Part model, mm, in its own coordinate system. Coordinates: 2 decimals unless noted, no trailing zeros. Loops run counter-clockwise (first coordinate to the right, second up) from the corner with the lowest first, then second, coordinate; pieces in that order, holes last. Notation, with made-up numbers: (60, -15.75) -> (76, -15.75) arc R20 cw to (76, -5.75) -> close; hole circle Ø7 at (-27.5, 27). An arc over 180 degrees is marked (long way). Use one line per item in the form item = value. Start each with the question number.
(1) Band-saw the part on B-B on z = 0.5. Give the cut face in (x, y) (3 decimals).
(2) Drill centre lines: L1, parallel to Y at x = 13.5, z = 0.25; L2, parallel to X at y = 26, z = 0.95; L3, parallel to Y at x = -27, z = 0.45. Where is each one in solid material? Low to high. Write a range as [from, to].
(3) Pin check, flat tips, straight feed: P1, Ø1.5, axis at x = -7, y = 9, coming from the -Z side; P2, Ø2, axis at x = -14.6, y = -25.4, coming from the +Z side. Stop position of each tip, or through.
(4) Band-saw the part on A-A on y = -25.5. Give the cut face in (x, z).
(5) Mould opens along X. For faces 1 (the flat face through (0, 29.769, 1)), 2 (the cylindrical face through (-15.755, 24.143, 0.773)), 3 (the cylindrical face through (14.5, 23.7, 0.8)), 4 (the flat face through (-29.529, -25.386, 0.773)) say: +X half, -X half, draft (parallel to the pull), parting line (faces both ways), or undercut.
Autodesk Inventor part; units mm, degrees
ref_plane "YZ Plane" through (0, 0, 0) normal (1, 0, 0) x (0, 1, 0)
ref_plane "XZ Plane" through (0, 0, 0) normal (0, 1, 0) x (-1, 0, 0)
ref_plane "XY Plane" through (0, 0, 0) normal (0, 0, 1) x (1, 0, 0)
sketch "Sketch1" plane through (0, 0, 0) normal (0, 0, 1) x (1, 0, 0)
  line L0 (-34.036, -29.7688) -> (34.036, -29.7688)
  line L1 (34.036, -29.7688) -> (34.036, 29.7688)
  line L2 (34.036, 29.7688) -> (-34.036, 29.7688)
  line L3 (-34.036, 29.7688) -> (-34.036, -29.7688)
  line L4 (-34.036, -29.7688) -> (34.036, 29.7688) construction
  line L5 (34.036, -29.7688) -> (-34.036, 29.7688) construction
  point P0 (0, 0)
  dimension "d0" = 68.072
  dimension "d1" = 59.5376
extrude "Extrusion1" add sketch "Sketch1" along normal blind 1.524
chamfer "Chamfer1" distance 8.89 angle 45 2 edges at (-34.036, -29.7688, 0.762) (34.036, -29.7688, 0.762)
sketch "Sketch3" plane through (0, 0, 0) normal (0, 0, -1) x (-1, 0, 0)
  circle A0 centre (-14.605, -25.4024) radius 1.7018
  circle A1 centre (14.605, -25.4024) radius 1.7018
  circle A2 centre (14.605, 25.3976) radius 1.7018
  circle A3 centre (-14.605, 25.3976) radius 1.7018
  point P0 (0, 0)
hole "Hole2" at (14.605, -25.4024, 0) at (-14.605, -25.4024, 0) at (-14.605, 25.3976, 0) at (14.605, 25.3976, 0) direction (0, 0, 1) diameter 3.4036 end through all
properties part number "DPLX_P031_VIPE Insulation Top" material "Polyethylene, High Density"
A:
q1.outline = (-34.036, -20.879) -> (-25.146, -29.769) -> (25.146, -29.769) -> (34.036, -20.879) -> (34.036, 29.769) -> (-34.036, 29.769) -> close; hole circle Ø3.404 at (-14.605, -25.402); hole circle Ø3.404 at (-14.605, 25.398); hole circle Ø3.404 at (14.605, -25.402); hole circle Ø3.404 at (14.605, 25.398)
q2.L1 = [-29.77, -26.7], [-24.11, 24.1], [26.69, 29.77]
q2.L2 = [-34.04, -16.2], [-13.01, 13.01], [16.2, 34.04]
q2.L3 = [-27.91, 29.77]
q3.P1 = 0
q3.P2 = through
q4.outline = (-29.41, 0) -> (-16.3, 0) -> (-16.3, 1.52) -> (-29.41, 1.52) -> close; (-12.91, 0) -> (12.91, 0) -> (12.91, 1.52) -> (-12.91, 1.52) -> close; (16.3, 0) -> (29.41, 0) -> (29.41, 1.52) -> (16.3, 1.52) -> close
q5.face_1 = draft
q5.face_2 = undercut
q5.face_3 = undercut
q5.face_4 = -X half
